from build123d import *

# Parameters (mm, degrees)
F1_DEPTH = 12
F2_R     = 6
F3_DEPTH = 32
F4_W     = 12
F4_H     = 27
F4_H_2   = 25
F5_DEPTH = 30.001


with BuildPart() as f1:
    # F0 (on Front) → F1 (new body)
    with BuildSketch(Plane.XZ):
        with BuildLine():
            Line((-16, 45), (-16, 0))
            ThreePointArc((-16, 0), (-11.313708, -11.313708), (0, -16))
            ThreePointArc((0, -16), (11.313708, -11.313708), (16, 0))
            Line((16, 0), (16, 45))
            Line((16, 45), (-16, 45))
        make_face()
        with BuildLine():
            ThreePointArc((0, -6), (-4.242641, -4.242641), (-6, 0))
            Line((-6, 0), (-6, 25))
            ThreePointArc((-6, 25), (-4.242641, 29.242641), (0, 31))
            ThreePointArc((0, 31), (4.242641, 29.242641), (6, 25))
            Line((6, 25), (6, 0))
            ThreePointArc((6, 0), (4.242641, -4.242641), (0, -6))
        make_face(mode=Mode.SUBTRACT)
    extrude(amount=F1_DEPTH)

    # F2 (on face) → F3 (join)
    with BuildSketch(Plane.YZ.offset(16)):
        with BuildLine():
            Line((0, 45), (0, 70))
            ThreePointArc((0, 70), (-25.323708, 80.882144), (-15.789474, 55.02079))
            ThreePointArc((-15.789474, 55.02079), (-13.098095, 53.779323), (-12, 51.026334))
            Line((-12, 51.026334), (-12, 45))
            Line((-12, 45), (0, 45))
        make_face()
        with Locations((-15, 70)):
            Circle(F2_R, mode=Mode.SUBTRACT)
    extrude(amount=-F3_DEPTH)

    # F4 (on face) → F5 (cut, through all)
    with BuildSketch(Plane(origin=(0, 0, 0), x_dir=(-1, 0, 0), z_dir=(0, 1, 0))):
        with Locations((0, 83.5)):
            Rectangle(F4_W, F4_H)
        with Locations((0, 57.5)):
            Rectangle(F4_W, F4_H_2)
    extrude(amount=-F5_DEPTH, mode=Mode.SUBTRACT)


solid = f1.part
Verification items for the finished model (mm, model axes). A direction names the side the tool comes from. Coordinates: 2 decimals unless noted, no trailing zeros. Write each loop counter-clockwise with the first axis right and the second up, starting at its lowest first coordinate (ties: lowest second). Pieces come first, ordered by that corner, then holes. Notation, with made-up numbers: M 28,14.5 L 52,14.5 A22 ccw 52,30.5 Z; hole C -19.75,84 d8. An arc over 180 degrees is marked long. Use CSV: the item, a comma, the result in double quotes.
Q1. Section check D-D, the plane y = -18. Enter the section's corners in (x, z).
Computed values:
outline,"M -16,55.3 L -6,55.3 L -6,64.8 L -16,64.8 Z; M -16,75.2 L -6,75.2 L -6,84.7 L -16,84.7 Z; M 6,55.3 L 16,55.3 L 16,64.8 L 6,64.8 Z; M 6,75.2 L 16,75.2 L 16,84.7 L 6,84.7 Z"
Q2. Set-up check for faces 5 (the flat face through (-16, -12, 53)), 6 (the flat face through (-6, -11, 65)), 7 (the flat face through (-7, -12, 18)), 8 (the cylindrical face through (11.07, -15.78, 75.95)), 9 (the flat face through (-6, -6, 12)): record each of +Z, -Z, +X, -X, +Y, -Y from which the full face is reachable in a straight line by a thin tool's end or side.
Computed values:
face 5,"+Z, -Z, -X, +Y, -Y"
face 6,"+Z, +Y, -Y"
face 7,"-Z, +X, -X, -Y"
face 8,"+X, -X"
face 9,"+Y, -Y"
Q3. Go/stop test with flat-tipped pins: P1, Ø12, axis at x = -12, y = -5.5, coming from the +Z side; P2, Ø10, axis at y = -7.5, z = -5.5, coming from the +X side; P3, Ø5, axis at x = -3, z = 45, coming from the +Y side; P4, Ø6, axis at x = 0.5, y = -7, coming from the +Z side. Record where each tip stops, or that it passes through.
Computed values:
P1,"z = 84.59"
P2,"x = 15.99"
P3,"y = 0"
P4,"z = 45"
Q4. Section check A-A, the plane z = 13.5. Enter the section's corners in (x, y), and give its area (3 significant figures).
Computed values:
outline,"M -16,-12 L -6,-12 L -6,0 L -16,0 Z; M 6,-12 L 16,-12 L 16,0 L 6,0 Z"
area,"240 mm²"
Q5. Mould release check, pull along Z, two halves, no side actions. Record for faces 1 (the flat face through (6, -6, 13)), 2 (the cylindrical face through (-10.93, -15.78, 75.95)), 3 (the flat face through (-7, 0, 26)), 4 (the flat face through (0, -6, 45)): pulls with the +Z half, pulls with the -Z half, needs draft (parallel to the pull), parting line crosses it, or undercut.
Computed values:
face 1,"undercut"
face 2,"undercut"
face 3,"needs draft"
face 4,"pulls with the +Z half"
Q6. Section check C-C, the plane y = -10. Enter the section's corners in (x, z), and give its area (3 significant figures).
Computed values:
outline,"M -16,0 A16 ccw 0,-16 A16 ccw 16,0 L 16,66.68 L 6,66.68 L 6,45 L -6,45 L -6,66.68 L -16,66.68 Z; M -16,73.32 L -6,73.32 L -6,84.14 L -16,84.14 Z; M 6,73.32 L 16,73.32 L 16,84.14 L 6,84.14 Z; hole M -6,0 A6 ccw 0,-6 A6 ccw 6,0 L 6,25 A6 ccw 0,31 A6 ccw -6,25 Z"
area,"2,080 mm²"
Q7. Thickness scan on line 1 along X through (y, z) = (-6.5, 20); line 2 along Y through (x, z) = (-12, 8); line 3 along Z through (x, y) = (-10.5, -15). Record the ranges inside material, lowest first. Write a range as [from, to].
Computed values:
line 1,"[-16, -6], [6, 16]"
line 2,"[-12, 0]"
line 3,"[54.9, 64], [76, 85]"
Q8. Section check B-B, the plane x = -1. Enter the section's corners in (y, z), and give its area (3 significant figures).
Computed values:
outline,"M -12,-15.97 L 0,-15.97 L 0,-5.92 L -12,-5.92 Z; M -12,30.92 L 0,30.92 L 0,45 L -12,45 Z"
area,"290 mm²"
